Part print with two shaded views. Sizes in mm from the minimum x, y, z corner. Round coordinates to 2 decimals unless told otherwise and drop trailing zeros. Loops run counter-clockwise (first coordinate to the right, second up) from the corner with the lowest first, then second, coordinate; pieces in that order, holes last.
(1) Cut at B-B on z = 0.8. Count the separate pieces of the cut face and the enclosed holes in it, then the cut area to 3 significant figures.
(2) Cut at C-C on y = 54. List the corners of the cut face in (x, z) (1 decimal).
(3) Probe probe 1 along Y at (x, z) = (117, 0.35); probe 2 along X at (y, z) = (51, 1.8) (1 decimal); probe 3 along X at (y, z) = (83, 0.9) (1 decimal). List the from-to ranges inside material, lowest first.
(4) Cut at D-D on x = 115. List the corners of the cut face in (y, z).
(5) Flat gauge pins, fed straight in: pin 1 (13 mm diameter, centred on x = 164.24, y = 51.85, fed in from -Z); pin 2 (8 mm diameter, centred on x = 70.91, y = 86.85, fed in from -Z). Where does each tip first touch, or does it go through?
(6) Cut at A-A on x = 70.5. List the corners of the cut face in (y, z).
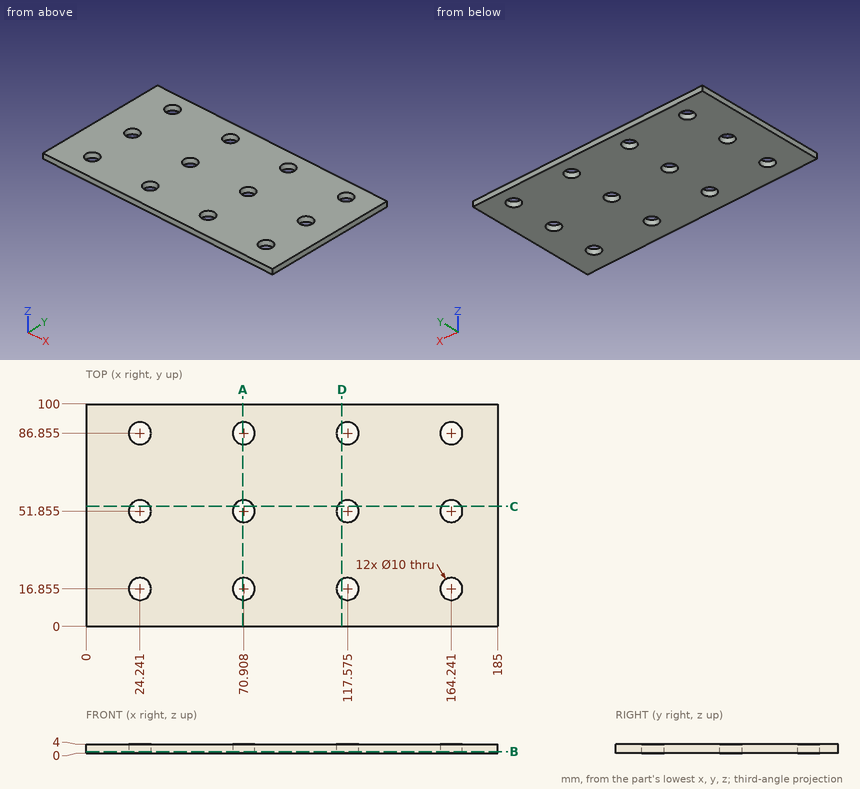
Final values:
1. separate pieces: 1
1. enclosed holes: 12
1. area: 17,600 mm2
2. outline: (0, 0) - (19.7, 0) - (19.7, 4) - (0, 4) - close; (28.8, 0) - (66.4, 0) - (66.4, 4) - (28.8, 4) - close; (75.4, 0) - (113.1, 0) - (113.1, 4) - (75.4, 4) - close; (122.1, 0) - (159.7, 0) - (159.7, 4) - (122.1, 4) - close; (168.8, 0) - (185, 0) - (185, 4) - (168.8, 4) - close
3. probe 1: y = 0 to 11.89, 21.82 to 46.89, 56.82 to 81.89, 91.82 to 100
3. probe 2: x = 0 to 19.3, 29.2 to 66, 75.8 to 112.6, 122.5 to 159.3, 169.2 to 185
3. probe 3: x = 0 to 21.1, 27.4 to 67.7, 74.1 to 114.4, 120.8 to 161.1, 167.4 to 185
4. outline: (0, 0) - (12.57, 0) - (12.57, 4) - (0, 4) - close; (21.14, 0) - (47.57, 0) - (47.57, 4) - (21.14, 4) - close; (56.14, 0) - (82.57, 0) - (82.57, 4) - (56.14, 4) - close; (91.14, 0) - (100, 0) - (100, 4) - (91.14, 4) - close
5. pin 1: stops at z = 0
5. pin 2: passes through
6. outline: (0, 0) - (11.87, 0) - (11.87, 4) - (0, 4) - close; (21.84, 0) - (46.87, 0) - (46.87, 4) - (21.84, 4) - close; (56.84, 0) - (81.87, 0) - (81.87, 4) - (56.84, 4) - close; (91.84, 0) - (100, 0) - (100, 4) - (91.84, 4) - close
